Check sheet for the modelled part. Datum: model origin and axes. Units: mm. Face numbers are marked on the shaded views. A direction names the side the tool comes from. Give positions to 0.01 mm unless a question says otherwise; leave off trailing zeros. Loops run counter-clockwise (first coordinate to the right, second up) from the corner with the lowest first, then second, coordinate; pieces in that order, holes last. Notation, with made-up numbers: (9, 27) - (58, 27) arc R35 cw to (58, 60) - close; hole circle Ø1 at (-35.75, 37.25). An arc over 180 degrees is marked (long way). Use one line per item in the form item = value.
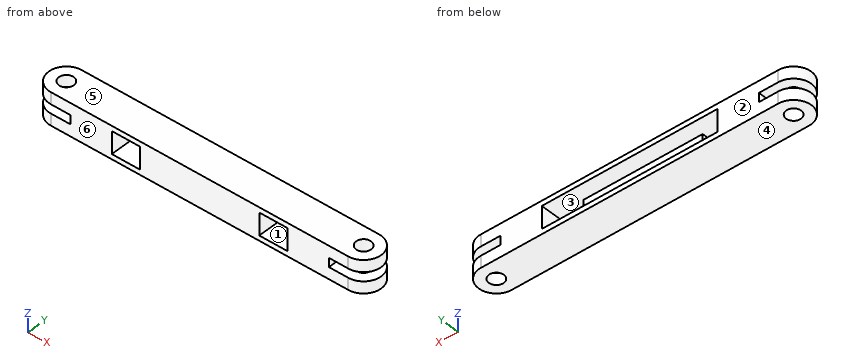
from build123d import *

# Parameters (mm, degrees)
SKETCH1_R           = 3.175
BOSS_EXTRUDE1_DEPTH = 5
SKETCH2_W           = 110.49
SKETCH2_H           = 15
BOSS_EXTRUDE2_DEPTH = 3.81
SKETCH5_R           = 3.175
BOSS_EXTRUDE3_DEPTH = 5
SKETCH6_W           = 75
SKETCH6_H           = 9.5
CUT_EXTRUDE1_DEPTH  = 6.5
SKETCH7_W           = 12
SKETCH7_H           = 9.5
CUT_EXTRUDE2_DEPTH  = 9.294


with BuildPart() as part:
    # Sketch1 → Boss-Extrude1 (new body)
    with BuildSketch(Plane.XY):
        with BuildLine():
            Line((-47.217391304, 7.923913043), (79.782608696, 7.923913043))
            ThreePointArc((79.782608696, 7.923913043), (87.282608696, 0.423913043), (79.782608696, -7.076086957))
            Line((79.782608696, -7.076086957), (-47.217391304, -7.076086957))
            ThreePointArc((-47.217391304, -7.076086957), (-54.717391304, 0.423913043), (-47.217391304, 7.923913043))
        make_face()
        with Locations((-47.217391304, 0.423913043)):
            Circle(SKETCH1_R, mode=Mode.SUBTRACT)
        with Locations((79.782608696, 0.423913043)):
            Circle(SKETCH1_R, mode=Mode.SUBTRACT)
    extrude(amount=BOSS_EXTRUDE1_DEPTH)

    # Sketch2 → Boss-Extrude2 (add)
    with BuildSketch(Plane.XY.offset(5)):
        with Locations((16.282608696, 0.423913043)):
            Rectangle(SKETCH2_W, SKETCH2_H)
    extrude(amount=BOSS_EXTRUDE2_DEPTH)

    # Sketch5 → Boss-Extrude3 (add)
    with BuildSketch(Plane.XY.offset(8.81)):
        with BuildLine():
            Line((-47.217391304, 7.923913043), (79.782608696, 7.923913043))
            ThreePointArc((79.782608696, 7.923913043), (87.282608696, 0.423913043), (79.782608696, -7.076086957))
            Line((79.782608696, -7.076086957), (-47.217391304, -7.076086957))
            ThreePointArc((-47.217391304, -7.076086957), (-54.717391304, 0.423913043), (-47.217391304, 7.923913043))
        make_face()
        with Locations((-47.217391304, 0.423913043)):
            Circle(SKETCH5_R, mode=Mode.SUBTRACT)
        with Locations((79.782608696, 0.423913043)):
            Circle(SKETCH5_R, mode=Mode.SUBTRACT)
    extrude(amount=BOSS_EXTRUDE3_DEPTH)

    # Sketch6 → Cut-Extrude1 (cut)
    with BuildSketch(Plane(origin=(0, 7.923913043, 0), x_dir=(1, 0, 0), z_dir=(0, 1, 0))):
        with Locations((16.282608696, -6.905)):
            Rectangle(SKETCH6_W, SKETCH6_H)
    extrude(amount=-CUT_EXTRUDE1_DEPTH, mode=Mode.SUBTRACT)

    # Sketch7 → Cut-Extrude2 (cut)
    with BuildSketch(Plane(origin=(0, 1.423913043, 0), x_dir=(1, 0, 0), z_dir=(0, 1, 0))):
        with Locations((-15.217391304, -6.905)):
            Rectangle(SKETCH7_W, SKETCH7_H)
        with Locations((47.782608696, -6.905)):
            Rectangle(SKETCH7_W, SKETCH7_H)
    extrude(amount=-CUT_EXTRUDE2_DEPTH, mode=Mode.SUBTRACT)


solid = part.part
Item 1: Gauge pin test, flat ends, axial feed: P1, Ø3, axis at x = 21, z = 7, coming from the +Y side; P2, Ø5.5, axis at x = 79.78, y = 0.42, coming from the -Z side; P3, Ø4, axis at y = 1.5, z = 7, coming from the +X side; P4, Ø1.9, axis at y = -2, z = 7.5, coming from the -X side. Record the tip position at first contact, or that the pin passes through.
Answer block:
P1 = 1.42
P2 = through
P3 = 87.28
P4 = -38.96
Item 2: Access from +Z, -Z, +X, -X, +Y, -Y to the whole of each face (thin tool, end or side, straight path). Record for the marked faces 1 and 2.
Answer block:
face_1 = +Y
face_2 = +Z, -Z, +X, -X, +Y
Item 3: Section check C-C on y = -5. Record the boundary of the cut face in (x, z) (3 decimals), then the cut area to 3 significant figures.
Answer block:
outline = (-52.397, 0) - (84.962, 0) - (84.962, 5) - (71.528, 5) - (71.528, 8.81) - (84.962, 8.81) - (84.962, 13.81) - (-52.397, 13.81) - (-52.397, 8.81) - (-38.962, 8.81) - (-38.962, 5) - (-52.397, 5) - close; hole (-21.217, 2.155) - (-9.217, 2.155) - (-9.217, 11.655) - (-21.217, 11.655) - close; hole (41.783, 2.155) - (53.783, 2.155) - (53.783, 11.655) - (41.783, 11.655) - close
area = 1,570 mm2
Item 4: Thickness scan on L1, parallel to Z at x = 35, y = 5.5 (3 decimals); L2, parallel to X at y = 5.25, z = 6; L3, parallel to X at y = 3.25, z = 2. Record the ranges inside material, lowest first.
Answer block:
L1 = 0 to 2.155, 11.655 to 13.81
L2 = -38.96 to -21.22, 53.78 to 71.53
L3 = -54.16 to -48.66, -45.77 to 78.34, 81.23 to 86.73
Item 5: Section check A-A on z = 7. Record the boundary of the cut face in (x, y).
Answer block:
outline = (-38.96, -7.08) - (-21.22, -7.08) - (-21.22, 7.92) - (-38.96, 7.92) - close; (-9.22, -7.08) - (41.78, -7.08) - (41.78, 1.42) - (-9.22, 1.42) - close; (53.78, -7.08) - (71.53, -7.08) - (71.53, 7.92) - (53.78, 7.92) - close
Item 6: Mould release check, pull along Z, two halves, no side actions. Record for the marked faces 3, 4, 5 and 6: released by +Z, released by -Z, zero draft, split by the parting line, or undercut.
Answer block:
face_3 = undercut
face_4 = released by -Z
face_5 = released by +Z
face_6 = zero draft
Item 7: Section check B-B on x = 11. Record the boundary of the cut face in (y, z) (3 decimals), then the cut area to 3 significant figures.
Answer block:
outline = (-7.076, 0) - (7.924, 0) - (7.924, 2.155) - (1.424, 2.155) - (1.424, 11.655) - (7.924, 11.655) - (7.924, 13.81) - (-7.076, 13.81) - close
area = 145 mm2
